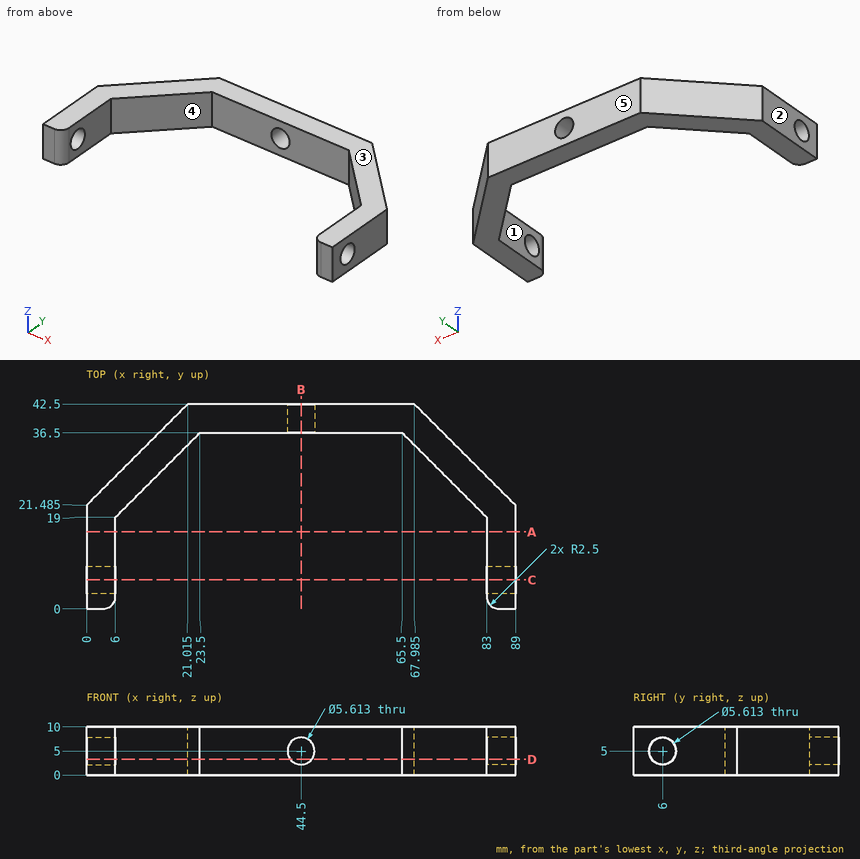
Drawing for the job (mm, zero at the part's lowest x, y, z). A direction names the side the tool comes from. Coordinates: 2 decimals unless noted, no trailing zeros. Write each loop counter-clockwise with the first axis right and the second up, starting at its lowest first coordinate (ties: lowest second). Pieces come first, ordered by that corner, then holes. Notation, with made-up numbers: (36, 51) -> (67, 51) arc R23 ccw to (67, 81) -> close; hole circle Ø4 at (89, 60.5). An arc over 180 degrees is marked (long way). One line per item, written item: value. Start each with the question number.
1) Slice it at C-C on y = 6. Write the cut outline in (x, z).
2) Slice it at A-A on y = 16. Write the cut outline in (x, z).
3) Slice it at D-D on z = 3.25. Write the cut outline in (x, y) (1 decimal), then the cut area to 3 significant figures.
4) Probe probe 1 along X at (y, z) = (4.5, 2.5); probe 2 along Z at (x, y) = (44.5, 39); probe 3 along Y at (x, z) = (50, 1.5). List the from-to ranges inside material, lowest first.
5) Slice it at B-B on x = 44.5. Write the cut outline in (y, z).
6) Flat gauge pins, fed straight in: pin 1 Ø12 at (x, y) = (33.5, 25) entering from -Z; pin 2 Ø5 at (x, z) = (54, 6) entering from -Y; pin 3 Ø1 at (y, z) = (38, 8.5) entering from -X (1 decimal); pin 4 Ø1 at (y, z) = (35, 2) entering from -X (1 decimal). Where does each tip first touch, or does it go through?
7) Pull direction X, two halves, no side cores. Call the marked faces 1, 2 and 3: +X half, -X half, draft (parallel to the pull), parting line (faces both ways), or undercut.
8) Which spindle directions (+Z, -Z, +X, -X, +Y, -Y) get a long thin tool onto all of the face, cutting with end or side? Do the marked faces 4 and 5. Say none if no direction does.
Answers follow:
1. outline: (0, 0) -> (6, 0) -> (6, 2.19) -> (0, 2.19) -> close; (0, 7.81) -> (6, 7.81) -> (6, 10) -> (0, 10) -> close; (83, 0) -> (89, 0) -> (89, 2.19) -> (83, 2.19) -> close; (83, 7.81) -> (89, 7.81) -> (89, 10) -> (83, 10) -> close
2. outline: (0, 0) -> (6, 0) -> (6, 10) -> (0, 10) -> close; (83, 0) -> (89, 0) -> (89, 10) -> (83, 10) -> close
3. outline: (0, 0) -> (3.5, 0) arc R2.5 ccw to (6, 2.5) -> (6, 3.8) -> (0, 3.8) -> close; (0, 8.2) -> (6, 8.2) -> (6, 19) -> (23.5, 36.5) -> (42.3, 36.5) -> (42.3, 42.5) -> (21, 42.5) -> (0, 21.5) -> close; (46.7, 36.5) -> (65.5, 36.5) -> (83, 19) -> (83, 8.2) -> (89, 8.2) -> (89, 21.5) -> (68, 42.5) -> (46.7, 42.5) -> close; (83, 2.5) arc R2.5 ccw to (85.5, 0) -> (89, 0) -> (89, 3.8) -> (83, 3.8) -> close
3. area: 755 mm2
4. probe 1: 0 to 6, 83 to 89
4. probe 2: 0 to 2.19, 7.81 to 10
4. probe 3: 36.5 to 42.5
5. outline: (36.5, 0) -> (42.5, 0) -> (42.5, 2.19) -> (36.5, 2.19) -> close; (36.5, 7.81) -> (42.5, 7.81) -> (42.5, 10) -> (36.5, 10) -> close
6. pin 1: through
6. pin 2: y = 36.5
6. pin 3: x = 16
6. pin 4: x = 13
7. face 1: undercut
7. face 2: -X half
7. face 3: draft
8. face 4: +Z, -Z, -Y
8. face 5: +Z, -Z, +X, -X, +Y
